The listing builds one solid part. Answer for the finished solid, in the listing's coordinates (mm). Round coordinates to 2 decimals unless told otherwise and drop trailing zeros. Write each loop counter-clockwise with the first axis right and the second up, starting at its lowest first coordinate (ties: lowest second). Pieces come first, ordered by that corner, then holes. Notation, with made-up numbers: (39, -17) - (96, -17) arc R28 cw to (96, 17) - close; hole circle Ø8 at (65, -37.75). An arc over 180 degrees is marked (long way). Use a Markdown table: item, result. Add a question column.
1) Find the intervals of material crossed by probe 1 along Y at (x, z) = (30.5, 0.4) (3 decimals); probe 2 along X at (y, z) = (-1, 2.75) (1 decimal); probe 3 along X at (y, z) = (-11, 0.9), in increasing order. Write a range as from..to.
2) A cutting plane is placed at C-C (x = 5). Give the vertices of the cut face in (y, z) (3 decimals).
3) Each of these flat-tipped pins is pushed along its axis until it touches: P1, Ø0.8, axis at y = 10.5, z = 0.5, coming from the -X side; P2, Ø1, axis at x = 88, z = 1, coming from the -Y side; P3, Ø3.5, axis at x = 88, y = 40.5, coming from the +Z side. Where does it stop, or does it pass through?
4) A cutting plane is placed at A-A (y = -44.5). Give the vertices of the cut face in (x, z) (1 decimal), then the cut area to 3 significant figures.
```python
from build123d import *

# Parameters (mm, degrees)
F1_DEPTH = 1.5875
F2_W     = 171.45
F2_H     = 174.625
F3_DEPTH = 1.5875
F4_W     = 136.525
F4_H     = 136.525
F5_DEPTH = 25.4


with BuildPart() as f1:
    # F0 (on Top) → F1 (new body)
    with BuildSketch(Plane.XY):
        with BuildLine():
            Line((87.3125, 88.9), (-87.3125, 88.9))
            Line((-87.3125, 88.9), (-88.519, 88.9))
            ThreePointArc((-88.519, 88.9), (-88.788408, 88.788408), (-88.9, 88.519))
            Line((-88.9, 88.519), (-88.9, 87.6935))
            ThreePointArc((-88.9, 87.6935), (-88.788408, 87.424092), (-88.519, 87.3125))
            Line((-88.519, 87.3125), (-87.3125, 87.3125))
            Line((-87.3125, 87.3125), (-87.3125, -85.725))
            Line((-87.3125, -85.725), (87.3125, -85.725))
            Line((87.3125, -85.725), (87.3125, 87.3125))
            Line((87.3125, 87.3125), (88.519, 87.3125))
            ThreePointArc((88.519, 87.3125), (88.788408, 87.424092), (88.9, 87.6935))
            Line((88.9, 87.6935), (88.9, 88.519))
            ThreePointArc((88.9, 88.519), (88.788408, 88.788408), (88.519, 88.9))
            Line((88.519, 88.9), (87.3125, 88.9))
        make_face()
    extrude(amount=F1_DEPTH)

    # F2 (on face) → F3 (join)
    with BuildSketch(Plane.XY.offset(1.5875)):
        with Locations((0, 1.5875)):
            Rectangle(F2_W, F2_H)
    extrude(amount=F3_DEPTH)

    # F4 (on face) → F5 (cut)
    with BuildSketch(Plane.XY.offset(3.175)):
        with Locations((0, 1.5875)):
            Rectangle(F4_W, F4_H)
    extrude(amount=-F5_DEPTH, mode=Mode.SUBTRACT)


solid = f1.part
```
Entries:
| question | item | result |
|---|---|---|
| 1 | probe 1 | y = -85.725..-66.675, 69.85..88.9 |
| 1 | probe 2 | x = -85.7..-68.3, 68.3..85.7 |
| 1 | probe 3 | x = -87.31..-68.26, 68.26..87.31 |
| 2 | outline | (-85.725, 0) - (-66.675, 0) - (-66.675, 3.175) - (-85.725, 3.175) - close; (69.85, 0) - (88.9, 0) - (88.9, 3.175) - (69.85, 3.175) - close |
| 3 | P1 | stops at x = -87.31 |
| 3 | P2 | stops at y = 87.31 |
| 3 | P3 | stops at z = 1.59 |
| 4 | outline | (-87.3, 0) - (-68.3, 0) - (-68.3, 3.2) - (-85.7, 3.2) - (-85.7, 1.6) - (-87.3, 1.6) - close; (68.3, 0) - (87.3, 0) - (87.3, 1.6) - (85.7, 1.6) - (85.7, 3.2) - (68.3, 3.2) - close |
| 4 | area | 116 mm² |
